Part model, mm, in its own coordinate system. A direction names the side the tool comes from. Give positions to 0.01 mm unless a question says otherwise; leave off trailing zeros. Write each loop counter-clockwise with the first axis right and the second up, starting at its lowest first coordinate (ties: lowest second). Pieces come first, ordered by that corner, then holes.
```python
from build123d import *

# Parameters (mm, degrees)
CHAMFER_SIZE = 1


with BuildPart() as part:
    # Sketch → Revolution (revolve)
    with BuildSketch(Plane.XY):
        Polygon((-102.5, 0), (-102.5, 25), (-82.5, 25), (-82.5, 5), (-20, 5), (-20, 25), (-12.5, 25), (-12.5, 0), (-12.5, -25), (-20, -25), (-20, -5), (-82.5, -5), (-82.5, -25), (-102.5, -25), align=None)
    revolve(axis=Axis((0, 0, 0), (0, 1, 0)))

    # Chamfer
    chamfer_edges = [part.edges().sort_by_distance(p)[0] for p in [
        (82.5, 25, 0),
        (102.5, -25, 0),
        (102.5, 25, 0),
        (20, 25, 0),
        (82.5, -25, 0),
        (20, -25, 0),
    ]]
    chamfer(chamfer_edges, length=CHAMFER_SIZE)


solid = part.part
```
1) 3-axis set-ups, long thin cutter, end or side, ignore diameter. For faces 5 (the face through (17.88, 14.37, -80.54)), 6 (the face through (-38, -25, -75)), 7 (the face through (17.88, -14.63, -80.54)): which of +Z, -Z, +X, -X, +Y, -Y reach the whole face in a straight line?
Answers follow:
face 5: +Y
face 6: +Z, -Z, +X, -X, -Y
face 7: -Y
2) Pin check, flat tips, straight feed: pin 1 Ø1 at (y, z) = (13, -38) entering from -X; pin 2 Ø1 at (y, z) = (9, -56.5) entering from +X; pin 3 Ø8 at (y, z) = (-13.5, -42.5) entering from +X; pin 4 Ø3 at (x, z) = (41, 72) entering from +Y. Stop position of each tip, or through.
Answers follow:
pin 1: stops at x = -95.39
pin 2: stops at x = 85.85
pin 3: stops at x = 94.99
pin 4: stops at y = 25
3) Wall check: L1, parallel to Z at x = 0, y = -11.5; L2, parallel to X at y = -22, z = -14; L3, parallel to X at y = -20.5, z = -13. Give the ranges that are in metal, low to high.
Answers follow:
L1: z = -102.5 to -82.5, -20 to -12.5, 12.5 to 20, 82.5 to 102.5
L2: x = -101.54 to -81.3, -14.28 to 14.28, 81.3 to 101.54
L3: x = -101.67 to -81.47, -15.2 to 15.2, 81.47 to 101.67
4) Saw through at A-A, the plane y = -18.5. Write the cut outline in (x, z).
Answers follow:
outline: circle Ø205 at (0, 0); circle Ø40 at (0, 0); hole circle Ø165 at (0, 0); hole circle Ø25 at (0, 0)
5) Two-plate mould, pull along Z, no slides. Class faces 1 (the face through (17, -5, -17)), 2 (the face through (-11.923, 0.35, 3.755)), 3 (the face through (4, -25, -12.4)), 4 (the face through (22.22, -0.336, -100.063)): +Z half, -Z half, draft (parallel to the pull), parting line (faces both ways), or undercut.
Answers follow:
face 1: undercut
face 2: undercut
face 3: draft
face 4: parting line
6) Saw through at B-B, the plane y = 1. Write the cut outline in (x, z), then the cut area to 3 significant figures.
Answers follow:
outline: circle Ø205 at (0, 0); hole circle Ø25 at (0, 0)
area: 32,500 mm2
